Verification items for the finished model (mm, model axes). Face numbers are marked on the shaded views. A direction names the side the tool comes from. Round coordinates to 2 decimals unless told otherwise and drop trailing zeros. Write each loop counter-clockwise with the first axis right and the second up, starting at its lowest first coordinate (ties: lowest second). Pieces come first, ordered by that corner, then holes. Notation, with made-up numbers: M 20,33 L 63,33 A23 cw 63,53 Z; hole C 17,82 d2. An arc over 180 degrees is marked long. One line per item, written item: value. Start each with the question number.
Item 1: Section check B-B, the plane y = -21. Record the cut outline in (x, z), then the cut area to 3 significant figures.
Item 2: Gauge pin test, flat ends, axial feed: pin 1 (7.5 mm diameter, centred on x = 70.5, y = -14.5, fed in from -Z); pin 2 (3.5 mm diameter, centred on x = 67, y = 21, fed in from +Z). Record the tip position at first contact, or that the pin passes through.
Item 3: Section check D-D, the plane z = 50.5. Record the cut outline in (x, y).
Item 4: Section check C-C, the plane x = 119. Record the cut outline in (y, z), then the cut area to 3 significant figures.
Item 5: Section check A-A, the plane y = -0.5. Record the cut outline in (x, z).
Item 6: Tool access check on the marked faces 1 and 2. Record the directions out of +Z, -Z, +X, -X, +Y, -Y that give a thin tool (end or side, any length) a straight path to the whole face; none if there is none.
Item 7: Draft check along Y on the marked faces 3, 4, 5 and 6. Enter one of: +Y half, -Y half, draft (parallel to the pull), parting line (faces both ways), or undercut.
Item 8: Thickness scan on probe 1 along X at (y, z) = (-2, 15); probe 2 along Y at (x, z) = (84, 57); probe 3 along X at (y, z) = (21, 77.9). Record the ranges inside material, lowest first. Write a range as from..to.
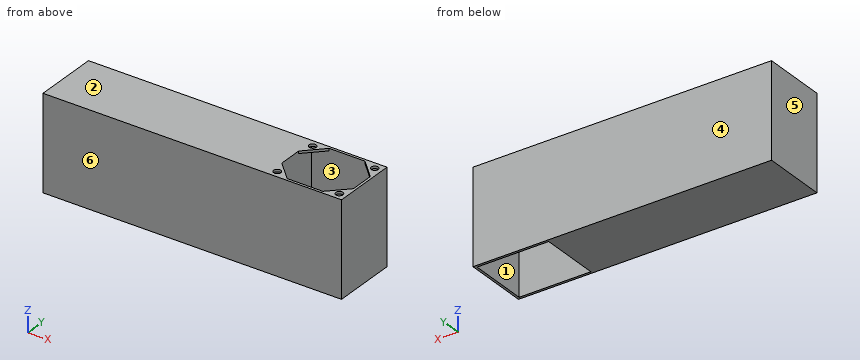
from build123d import *

# Parameters (mm, degrees)
STRUCTURESKETCH002_W      = 250
STRUCTURESKETCH002_H      = 54
MAINSTRUCTURE002_DEPTH    = 79
OBJ1           = 3
CENTERPOCKET002_DEPTH     = 79
OBJ2       = 60
OBJ3       = 50
OBJ4 = 77


with BuildPart() as part:
    # StructureSketch002 → MainStructure002 (new body)
    with BuildSketch(Plane.XY):
        Rectangle(STRUCTURESKETCH002_W, STRUCTURESKETCH002_H)
    extrude(amount=MAINSTRUCTURE002_DEPTH)

    with BuildSketch(Plane(origin=(93, 0, 0), x_dir=(1, 0, 0), z_dir=(0, 0, 1))):
        with Locations((-26, 21)):
            Circle(OBJ1)
        with Locations((26, 21)):
            Circle(OBJ1)
        with Locations((26, -21)):
            Circle(OBJ1)
        with Locations((-26, -21)):
            Circle(OBJ1)
        Polygon((-15, 25), (15, 25), (30, 10), (30, -10), (15, -25), (-15, -25), (-30, -10), (-30, 10), align=None)
    extrude(amount=CENTERPOCKET002_DEPTH, mode=Mode.SUBTRACT)

    with BuildSketch(Plane(origin=(93, 0, 0), x_dir=(1, 0, 0), z_dir=(0, 0, 1))):
        Rectangle(OBJ2, OBJ3)
    extrude(amount=OBJ4, mode=Mode.SUBTRACT)


solid = part.part
Response values:
1. outline: M -125,0 L 63,0 L 63,77 L 64,77 L 64,79 L -125,79 Z; M 70,77 L 74,77 L 74,79 L 70,79 Z; M 112,77 L 116,77 L 116,79 L 112,79 Z; M 122,77 L 123,77 L 123,0 L 125,0 L 125,79 L 122,79 Z
1. area: 15,000 mm2
2. pin 1: stops at z = 77
2. pin 2: passes through
3. outline: M -125,-27 L 125,-27 L 125,27 L -125,27 Z; hole M 63,-25 L 123,-25 L 123,25 L 63,25 Z
4. outline: M -27,0 L -25,0 L -25,77 L -24,77 L -24,79 L -27,79 Z; M -18,77 L -14,77 L -14,79 L -18,79 Z; M 14,77 L 18,77 L 18,79 L 14,79 Z; M 24,77 L 25,77 L 25,0 L 27,0 L 27,79 L 24,79 Z
4. area: 336 mm2
5. outline: M -125,0 L 63,0 L 63,79 L -125,79 Z; M 123,0 L 125,0 L 125,79 L 123,79 Z
6. face 1: -Z
6. face 2: +Z, +X, -X, +Y, -Y
7. face 3: undercut
7. face 4: +Y half
7. face 5: draft
7. face 6: -Y half
8. probe 1: x = -125..63, 123..125
8. probe 2: y = -27..-25, 25..27
8. probe 3: x = -125..64, 70..74, 112..116, 122..125
